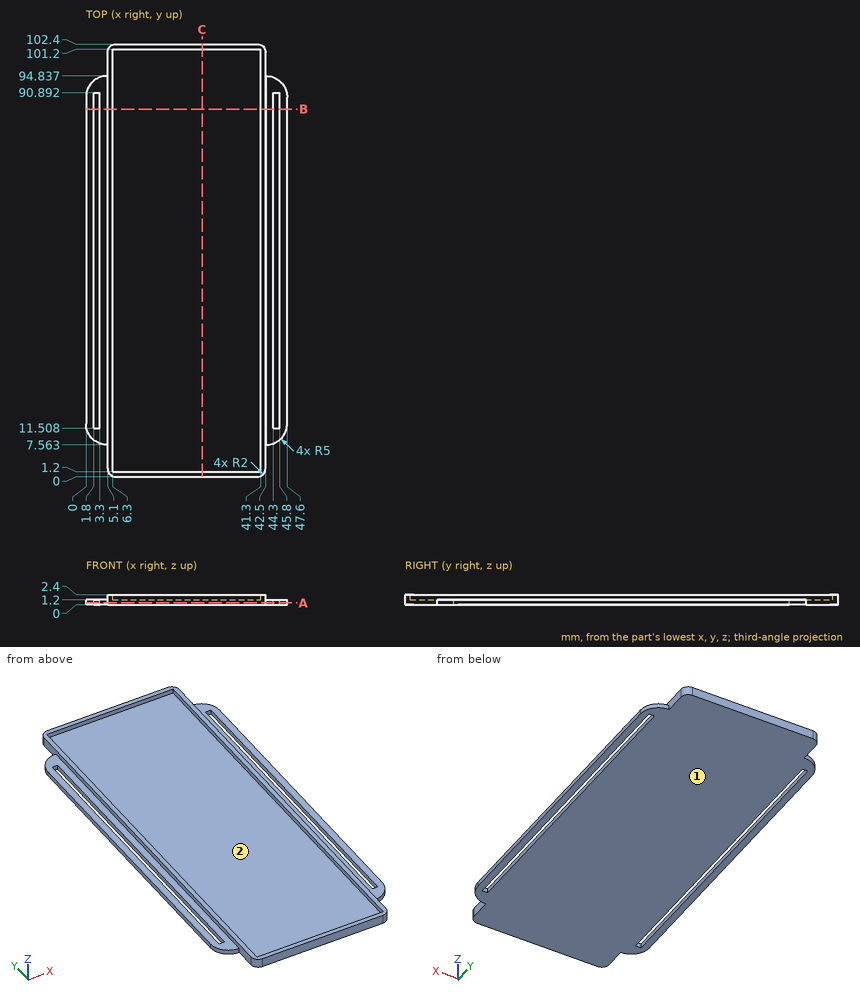
The drawing under review shows one solid part. Ordinate dimensions are in mm from its lowest x, y, z. Round coordinates to 2 decimals unless told otherwise and drop trailing zeros. Write each loop counter-clockwise with the first axis right and the second up, starting at its lowest first coordinate (ties: lowest second). Pieces come first, ordered by that corner, then holes. Notation, with made-up numbers: (-15.75, -7.75) -> (-10.75, -7.75) arc R9 cw to (-10.75, 1.25) -> close; hole circle Ø8 at (-5, 65). An arc over 180 degrees is marked (long way). One line per question, with ' | ' between items.
(1) Wall thickness on line 1 (X direction, y = 89, z = 0.2); line 2 (X direction, y = 90, z = 1.65); line 3 (Y direction, x = 34, z = 1.9): over which ranges is each line inside the solid? List them lowest first. Write a range as [from, to].
Result sheet:
line 1: [0, 1.8], [3.3, 44.3], [45.8, 47.6] | line 2: [5.1, 6.3], [41.3, 42.5] | line 3: [0, 1.2], [101.2, 102.4]
(2) Draft analysis for pull direction X (two halves, no side actions). For the marked faces 1 and 2, state which applies: released by +X, released by -X, zero draft, split by the parting line, or undercut.
Result sheet:
face 1: zero draft | face 2: undercut
(3) Take a section at A-A, the plane z = 0.5. State the section outline as (x, y) points, and give its area (3 significant figures).
Result sheet:
outline: (0, 12.56) arc R5 ccw to (5, 7.56) -> (5.1, 7.56) -> (5.1, 2) arc R2 ccw to (7.1, 0) -> (40.5, 0) arc R2 ccw to (42.5, 2) -> (42.5, 7.56) -> (42.6, 7.56) arc R5 ccw to (47.6, 12.56) -> (47.6, 89.84) arc R5 ccw to (42.6, 94.84) -> (42.5, 94.84) -> (42.5, 100.4) arc R2 ccw to (40.5, 102.4) -> (7.1, 102.4) arc R2 ccw to (5.1, 100.4) -> (5.1, 94.84) -> (5, 94.84) arc R5 ccw to (0, 89.84) -> close; hole (1.8, 11.51) -> (3.3, 11.51) -> (3.3, 90.89) -> (1.8, 90.89) -> close; hole (44.3, 11.51) -> (45.8, 11.51) -> (45.8, 90.89) -> (44.3, 90.89) -> close | area: 4,460 mm2
(4) Take a section at B-B, the plane y = 87. State the section outline as (x, z) points.
Result sheet:
outline: (0, 0) -> (1.8, 0) -> (1.8, 1.2) -> (0, 1.2) -> close; (3.3, 0) -> (44.3, 0) -> (44.3, 1.2) -> (42.5, 1.2) -> (42.5, 2.4) -> (41.3, 2.4) -> (41.3, 1.2) -> (6.3, 1.2) -> (6.3, 2.4) -> (5.1, 2.4) -> (5.1, 1.2) -> (3.3, 1.2) -> close; (45.8, 0) -> (47.6, 0) -> (47.6, 1.2) -> (45.8, 1.2) -> close
(5) Insertion check: P1, Ø0.6, axis at y = 72, z = 2, coming from the -X side; P2, Ø6, axis at x = 25.5, y = 14.5, coming from the -Z side; P3, Ø1.3, axis at x = 3, z = 0.5, coming from the -Y side; P4, Ø1, axis at y = 73.5, z = 2, coming from the +X side. Each pin has a flat end and moves straight along its axis. Give the tip position at first contact, or say it passes through.
Result sheet:
P1: x = 5.1 | P2: z = 0 | P3: y = 7.75 | P4: x = 42.5
(6) Take a section at C-C, the plane x = 27.5. State the section outline as (y, z) points.
Result sheet:
outline: (0, 0) -> (102.4, 0) -> (102.4, 2.4) -> (101.2, 2.4) -> (101.2, 1.2) -> (1.2, 1.2) -> (1.2, 2.4) -> (0, 2.4) -> close
